Check sheet for the drawn part. Datum: minimum x, y, z corner. Units: mm. A direction names the side the tool comes from. Coordinates: 2 decimals unless noted, no trailing zeros. Order: outer loops, then holes, each group sorted by start corner. A loop starts at its lowest first (then second) coordinate and runs counter-clockwise, first axis right, second up.
Q1. Thickness scan on line 1 (Y direction, x = 30, z = 3.6); line 2 (X direction, y = 10, z = 35); line 3 (Z direction, x = 33, y = 10). Record the ranges inside material, lowest first.
Q2. Depth check by flat-ended pin: P1, Ø10, axis at x = 50, y = 17.5, coming from the -Z side; P2, Ø10, axis at x = 20.5, y = 10, coming from the +Z side; P3, Ø10, axis at x = 10.5, y = 14.5, coming from the +Z side (1 decimal). Enter the tip coordinate at first touch or a pass-through.
Q3. Cross-section at A-A, the plane z = 37. Record the boundary of the cut face in (x, y), and give its area (3 significant figures).
Q4. Set-up check for the marked faces 5 and 6: record each of +Z, -Z, +X, -X, +Y, -Y from which the full face is reachable in a straight line by a thin tool's end or side.
Q5. Cross-section at B-B, the plane x = 30. Record the boundary of the cut face in (y, z).
Q6. Draft check along X on the marked faces 1, 2, 3 and 4. Enter one of: pulls with the +X half, pulls with the -X half, needs draft (parallel to the pull), parting line crosses it, or undercut.
Q7. Cross-section at D-D, the plane z = 55. Record the boundary of the cut face in (x, y).
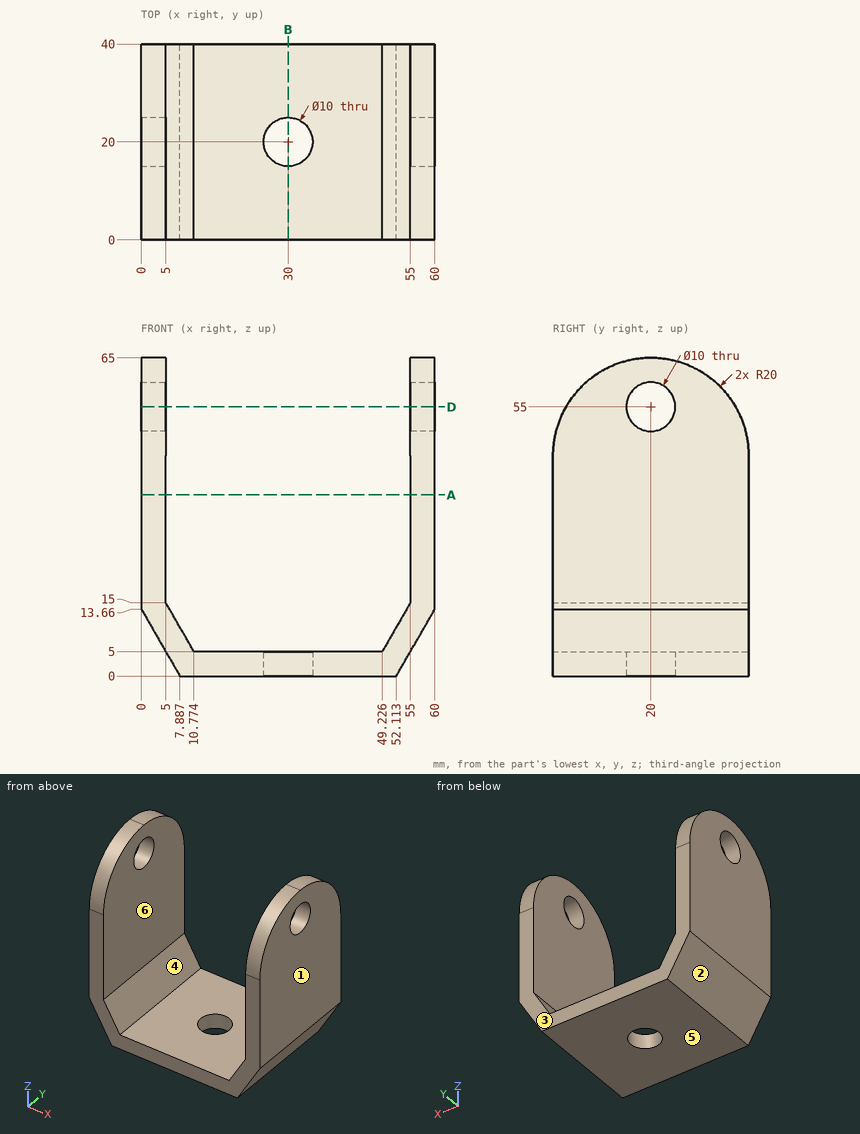
Check values:
1. line 1: y = 0 to 15, 25 to 40
1. line 2: x = 0 to 5, 55 to 60
1. line 3: z = 0 to 5
2. P1: stops at z = 0
2. P2: stops at z = 5
2. P3: stops at z = 14.1
3. outline: (0, 0) - (5, 0) - (5, 40) - (0, 40) - close; (55, 0) - (60, 0) - (60, 40) - (55, 40) - close
3. area: 400 mm2
4. face 5: -Z, +X, -X, +Y, -Y
4. face 6: +Z, +Y, -Y
5. outline: (0, 0) - (15, 0) - (15, 5) - (0, 5) - close; (25, 0) - (40, 0) - (40, 5) - (25, 5) - close
6. face 1: pulls with the +X half
6. face 2: pulls with the -X half
6. face 3: needs draft
6. face 4: undercut
7. outline: (0, 2.68) - (5, 2.68) - (5, 15) - (0, 15) - close; (0, 25) - (5, 25) - (5, 37.32) - (0, 37.32) - close; (55, 2.68) - (60, 2.68) - (60, 15) - (55, 15) - close; (55, 25) - (60, 25) - (60, 37.32) - (55, 37.32) - close
